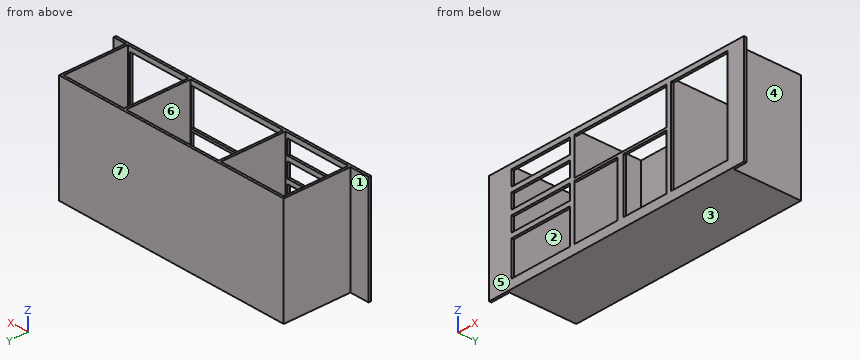
from build123d import *

# Parameters (mm, degrees)
F0_W     = 520
F0_H     = 494
F0_W_2   = 768
F0_W_3   = 500
F1_DEPTH = 820
F2_W     = 484
F2_H     = 114
F2_H_2   = 264
F2_W_2   = 357
F2_H_3   = 414
F3_DEPTH = 50
F4_W     = 1835.1259900331
F4_H     = 504.2004961409
F5_DEPTH = 18


# Not quite as in the source:
# - a feature names something its author has since deleted; it is built from what else it names


with BuildPart() as f1:
    # F0 (on Top) → F1 (new body)
    with BuildSketch(Plane.XY):
        Polygon((-150, 0), (0, 0), (1860, 0), (1960, 0), (1960, 18), (1860, 18), (1860, 530), (0, 530), (0, 18), (-150, 18), align=None)
        with Locations((278, 265)):
            Rectangle(F0_W, F0_H, mode=Mode.SUBTRACT)
        with Locations((940, 265)):
            Rectangle(F0_W_2, F0_H, mode=Mode.SUBTRACT)
        with Locations((1592, 265)):
            Rectangle(F0_W_3, F0_H, mode=Mode.SUBTRACT)
    extrude(amount=-F1_DEPTH)

    # F2 (on face) → F3 (cut)
    with BuildSketch(Plane.XZ):
        with Locations((278, -95)):
            Rectangle(F2_W, F2_H)
        with Locations((278, -245)):
            Rectangle(F2_W, F2_H)
        with Locations((278, -395)):
            Rectangle(F2_W, F2_H)
        with Locations((278, -620)):
            Rectangle(F2_W, F2_H_2)
        Polygon((556, -257.2889821529), (556, -320), (1320, -320), (1320, -38), (913, -38), (556, -38), align=None)
        with Locations((1141.5, -545)):
            Rectangle(F2_W_2, F2_H_3)
        Polygon((1572, -38), (1356, -38), (1356, -752), (1572, -752), (1608, -752), (1824, -752), (1824, -38), (1608, -38), align=None)
        Polygon((913, -338), (556, -338), (556, -407.2889821529), (556, -557.2889821529), (556, -752), (913, -752), align=None)
    extrude(amount=-F3_DEPTH, mode=Mode.SUBTRACT)

    # F4 (on face) → F5 (join)
    with BuildSketch(Plane(origin=(0, 0, -820), x_dir=(1, 0, 0), z_dir=(0, 0, -1))):
        with Locations((924.4370049834, -259.8997519296)):
            Rectangle(F4_W, F4_H)
    extrude(amount=-F5_DEPTH)


solid = f1.part
Design review of the part built by this model. Coordinates are the model's own, in mm. Face numbers are marked on the shaded views. A direction names the side the tool comes from. Give positions to 0.01 mm unless a question says otherwise; leave off trailing zeros. Write each loop counter-clockwise with the first axis right and the second up, starting at its lowest first coordinate (ties: lowest second). Pieces come first, ordered by that corner, then holes. Notation, with made-up numbers: M -13,46 L 40,46 A7 ccw 40,58 Z; hole C -39.75,73 d9. An arc over 180 degrees is marked long. Return JSON: item names as keys, results as strings. Group by question number.
Item 1: Wall thickness on line 1 along X through (y, z) = (244, -612); line 2 along Y through (x, z) = (1835, -259); line 3 along Y through (x, z) = (643, -271.5): over which ranges is each line inside the solid? List them lowest first.
Item 2: The part is to be moulded in two halves that separate along Y. For the marked faces 5, 6 and 7, say which applies: pulls with the +Y half, pulls with the -Y half, needs draft (parallel to the pull), parting line crosses it, or undercut.
Item 3: Clearance check with flat-ended pins moving along their axes: pin 1 Ø4 at (y, z) = (222, -128.5) entering from -X; pin 2 Ø1 at (x, y) = (1678.5, 293) entering from +Z; pin 3 Ø6 at (y, z) = (466, -466) entering from +X. State where each tip first meets the part, or that it passes through.
Item 4: Take a section at A-A (x = 1382). Give the boundary of the cut face in (y, z).
Item 5: Take a section at C-C (x = 1031). Give the boundary of the cut face in (y, z).
Item 6: Tool access review of the marked faces 1, 2, 3 and 4: name each direction out of +Z, -Z, +X, -X, +Y, -Y from which nothing blocks a thin tool from reaching the whole face with its end or side.
Return value:
{
 "1": {"line 1": "x = 0 to 18, 538 to 556, 1324 to 1342, 1842 to 1860", "line 2": "y = 0 to 18, 512 to 530", "line 3": "y = 512 to 530"},
 "2": {"face 5": "pulls with the -Y half", "face 6": "undercut", "face 7": "pulls with the +Y half"},
 "3": {"pin 1": "stops at x = 0", "pin 2": "stops at z = -802", "pin 3": "stops at x = 1860"},
 "4": {"outline": "M 0,-820 L 530,-820 L 530,0 L 512,0 L 512,-802 L 18,-802 L 18,-752 L 0,-752 Z; M 0,-38 L 18,-38 L 18,0 L 0,0 Z"},
 "5": {"outline": "M 0,-820 L 530,-820 L 530,0 L 512,0 L 512,-802 L 18,-802 L 18,-752 L 0,-752 Z; M 0,-338 L 18,-338 L 18,-320 L 0,-320 Z; M 0,-38 L 18,-38 L 18,0 L 0,0 Z"},
 "6": {"face 1": "+Z, -Z, -X, +Y", "face 2": "+Z", "face 3": "-Z, +X, -X, +Y, -Y", "face 4": "+Z, -Z, +X, +Y"}
}
